Build history of the part. All positions in model axes, mm. A direction names the side the tool comes from. Give positions to 0.01 mm unless a question says otherwise; leave off trailing zeros. Order: outer loops, then holes, each group sorted by start corner. A loop starts at its lowest first (then second) coordinate and runs counter-clockwise, first axis right, second up. Notation, with made-up numbers: M -10,60 L -5,60 A18 ccw -5,85 Z; hole C 8.25,-35.75 d9. An arc over 180 degrees is marked long. Use CSV: the item, a comma, the result in double quotes. Start each with the question number.
Item 1: Pin check, flat tips, straight feed: P1, Ø4, axis at x = -22, z = -60.5, coming from the -Y side; P2, Ø6, axis at x = 15, y = 40, coming from the -Z side; P3, Ø0.6, axis at x = 64, z = 46.5, coming from the +Y side; P4, Ø19, axis at y = 17, z = -42, coming from the -X side. Stop position of each tip, or through.
Item 2: Two-plate mould, pull along Z, no slides. Class faces 1 (the cylindrical face through (63.668, 32.972, -62.917)), 2 (the flat face through (2, 26, 78)), 3 (the flat face through (2, 51.18, -11)): pulls with the +Z half, pulls with the -Z half, needs draft (parallel to the pull), parting line crosses it, or undercut.
Item 3: Which spindle directions (+Z, -Z, +X, -X, +Y, -Y) get a long thin tool onto all of the face, cutting with end or side? Do faces 4 (the flat face through (-46.25, 26, -8)), 5 (the flat face through (50.75, 26, -8)), 6 (the flat face through (2, 26, -97.26)), 7 (the cylindrical face through (63.668, 31.413, 50.789)). Say none if no direction does.
Item 4: Wall check: line 1 along X through (y, z) = (37.5, -30); line 2 along Y through (x, z) = (63.5, 54.07); line 3 along Z through (x, y) = (-9, 33). Give the ranges that are in metal, low to high.
Item 5: Band-saw the part on A-A on x = -31.25. Write the cut outline in (y, z), plus the area to 3 significant figures.
Item 6: Band-saw the part on B-B on z = -65.46. Write the cut outline in (x, y).
Item 7: Band-saw the part on D-D on x = 42. Write the cut outline in (y, z).
Item 8: Band-saw the part on C-C on y = 6. Write the cut outline in (x, z).
from build123d import *

# Parameters (mm, degrees)
SKETCH1_W        = 128.5
SKETCH1_H        = 212
SKETCH1_R        = 3.15
SKETCH1_R_2      = 2.215
BASE_DEPTH       = 1.18
SKETCH4_W        = 97
SKETCH4_H        = 175.26
CAPACITORS_DEPTH = 50
SKETCH2_W        = 1.18
SKETCH2_H        = 60.3
SKETCH2_H_2      = 53.1
TABS_DEPTH       = 38
TAB_HOLES_REACH  = 130.5
SKETCH3_R        = 3.44
SKETCH3_R_2      = 3.45


with BuildPart() as part:
    # Sketch1 → Base (new body)
    with BuildSketch(Plane(origin=(0, 0, 0), x_dir=(1, 0, 0), z_dir=(0, 1, 0))):
        Rectangle(SKETCH1_W, SKETCH1_H)
        with Locations((-55.25, -78)):
            Circle(SKETCH1_R, mode=Mode.SUBTRACT)
        with Locations((-31.25, -102.185)):
            Circle(SKETCH1_R_2, mode=Mode.SUBTRACT)
    extrude(amount=BASE_DEPTH)

    # Sketch4 → Capacitors (add)
    with BuildSketch(Plane(origin=(0, 1.18, 0), x_dir=(1, 0, 0), z_dir=(0, 1, 0))):
        with Locations((2.25, 9.63)):
            Rectangle(SKETCH4_W, SKETCH4_H)
    extrude(amount=CAPACITORS_DEPTH)

    # Sketch2 → Tabs (add)
    with BuildSketch(Plane(origin=(0, 1.18, 0), x_dir=(1, 0, 0), z_dir=(0, 1, 0))):
        with Locations((63.66, -40.85)):
            Rectangle(SKETCH2_W, SKETCH2_H)
        with Locations((63.66, 48.35)):
            Rectangle(SKETCH2_W, SKETCH2_H_2)
    extrude(amount=TABS_DEPTH)

    # Sketch3 → Tab Holes (cut, up to next)
    with BuildSketch(Plane(origin=(64.25, 0, 0), x_dir=(0, 0, -1), z_dir=(1, 0, 0)), mode=Mode.PRIVATE) as tab_holes_sk1:
        with Locations((-54.07, 30.38)):
            Circle(SKETCH3_R)
    tab_holes_tool1 = extrude(tab_holes_sk1.sketch, amount=-TAB_HOLES_REACH, mode=Mode.PRIVATE) & part.part
    add(tab_holes_tool1.solids().sort_by_distance((64.25, 30.38, 54.07))[0], mode=Mode.SUBTRACT)
    # Sketch3 → Tab Holes (cut, up to next)
    with BuildSketch(Plane(origin=(64.25, 0, 0), x_dir=(0, 0, -1), z_dir=(1, 0, 0)), mode=Mode.PRIVATE) as tab_holes_sk2:
        with Locations((65.46, 30.64)):
            Circle(SKETCH3_R_2)
    tab_holes_tool2 = extrude(tab_holes_sk2.sketch, amount=-TAB_HOLES_REACH, mode=Mode.PRIVATE) & part.part
    add(tab_holes_tool2.solids().sort_by_distance((64.25, 30.64, -65.46))[0], mode=Mode.SUBTRACT)


solid = part.part
Model answer:
1,P1,"stops at y = 0"
1,P2,"stops at z = -97.26"
1,P3,"stops at y = 39.18"
1,P4,"stops at x = -46.25"
2,face 1,"undercut"
2,face 2,"pulls with the +Z half"
2,face 3,"needs draft"
3,face 4,"+Z, -Z, -X, +Y"
3,face 5,"+Z, -Z, +Y"
3,face 6,"-Z, +X, -X, +Y"
3,face 7,"+X"
4,line 1,"x = -46.25 to 50.75, 63.07 to 64.25"
4,line 2,"y = 0 to 26.94, 33.82 to 39.18"
4,line 3,"z = -97.26 to 78"
5,outline,"M 0,-106 L 1.18,-106 L 1.18,-97.26 L 51.18,-97.26 L 51.18,78 L 1.18,78 L 1.18,99.97 L 0,99.97 Z; M 0,104.4 L 1.18,104.4 L 1.18,106 L 0,106 Z"
5,area,"9,010 mm^2"
6,outline,"M -64.25,0 L 64.25,0 L 64.25,27.19 L 63.07,27.19 L 63.07,1.18 L 50.75,1.18 L 50.75,51.18 L -46.25,51.18 L -46.25,1.18 L -64.25,1.18 Z; M 63.07,34.09 L 64.25,34.09 L 64.25,39.18 L 63.07,39.18 Z"
7,outline,"M 0,-106 L 1.18,-106 L 1.18,-97.26 L 51.18,-97.26 L 51.18,78 L 1.18,78 L 1.18,106 L 0,106 Z"
8,outline,"M -46.25,-97.26 L 50.75,-97.26 L 50.75,78 L -46.25,78 Z; M 63.07,-74.9 L 64.25,-74.9 L 64.25,-21.8 L 63.07,-21.8 Z; M 63.07,10.7 L 64.25,10.7 L 64.25,71 L 63.07,71 Z"
